Verification items for the finished model (mm, model axes). A direction names the side the tool comes from. Round coordinates to 2 decimals unless told otherwise and drop trailing zeros. Write each loop counter-clockwise with the first axis right and the second up, starting at its lowest first coordinate (ties: lowest second). Pieces come first, ordered by that corner, then holes. Notation, with made-up numbers: (53, -24) - (107, -24) arc R20 ccw to (107, 10) - close; hole circle Ø6 at (12.25, -7). An arc over 180 degrees is marked (long way). Answer as a JSON object with one key per item and string values.
```python
from build123d import *

# Parameters (mm, degrees)
SKETCH1_R           = 7
BOSS_EXTRUDE1_DEPTH = 4
SKETCH2_R           = 7
SKETCH2_R_2         = 5
BOSS_EXTRUDE2_DEPTH = 10
BOSS_EXTRUDE3_DEPTH = 10
BOSS_EXTRUDE4_DEPTH = 9
FILLET3_R           = 1.35
CHAMFER1_SIZE       = 2.7
SKETCH7_R           = 1.5
CUT_EXTRUDE1_DEPTH  = 10
FILLET4_R           = 2
SKETCH8_R           = 0.5
CUT_EXTRUDE2_DEPTH  = 25.534299997


# Some blends are built 0.0001 mm under size
with BuildPart() as part:
    # Sketch1 → Boss-Extrude1 (new body)
    with BuildSketch(Plane.XY):
        Circle(SKETCH1_R)
    extrude(amount=BOSS_EXTRUDE1_DEPTH)

    # Sketch2 → Boss-Extrude2 (add)
    with BuildSketch(Plane.XY.offset(4)):
        Circle(SKETCH2_R)
        Circle(SKETCH2_R_2, mode=Mode.SUBTRACT)
    extrude(amount=BOSS_EXTRUDE2_DEPTH)

    # Sketch3 → Boss-Extrude3 (add)
    with BuildSketch(Plane.XY.offset(4)):
        with BuildLine():
            Line((-1.35, 4.814301611), (-1.35, -4.814301611))
            ThreePointArc((-1.35, -4.814301611), (-5, 0), (-1.35, 4.814301611))
        make_face()
        with BuildLine():
            Line((1.35, 4.814301611), (1.35, -4.814301611))
            ThreePointArc((1.35, -4.814301611), (5, 0), (1.35, 4.814301611))
        make_face()
    extrude(amount=BOSS_EXTRUDE3_DEPTH)

    # Sketch4 → Boss-Extrude4 (add)
    with BuildSketch(Plane(origin=(0, 0, 0), x_dir=(-1, 0, 0), z_dir=(0, 0, -1))):
        with BuildLine():
            Line((2.05, 0), (4.242640687, 0))
            Line((4.242640687, 0), (10.242640687, 0))
            Line((10.242640687, 0), (10.242640687, -1.5))
            Line((10.242640687, -1.5), (4.242640687, -1.5))
            ThreePointArc((4.242640687, -1.5), (0, -4.5), (-4.242640687, -1.5))
            Line((-4.242640687, -1.5), (-10.242640687, -1.5))
            Line((-10.242640687, -1.5), (-10.242640687, 0))
            Line((-10.242640687, 0), (-4.242640687, 0))
            Line((-4.242640687, 0), (-2.05, 0))
            ThreePointArc((-2.05, 0), (0, -2.05), (2.05, 0))
        make_face()
    extrude(amount=BOSS_EXTRUDE4_DEPTH)

    # Fillet3
    fillet3_edges = [part.edges().sort_by_distance(p)[0] for p in [
        (-1.35, 4.814301611, 9),
    ]]
    fillet(fillet3_edges, radius=FILLET3_R)
    fillet3_2_edges = [part.edges().sort_by_distance(p)[0] for p in [
        (1.35, 4.814301611, 9),
    ]]
    fillet(fillet3_2_edges, radius=FILLET3_R - 0.0001)  # a hair under: the kernel refuses the full size
    fillet3_3_edges = [part.edges().sort_by_distance(p)[0] for p in [
        (1.35, -4.814301611, 9),
    ]]
    fillet(fillet3_3_edges, radius=FILLET3_R)
    fillet3_4_edges = [part.edges().sort_by_distance(p)[0] for p in [
        (-1.35, -4.814301611, 9),
    ]]
    fillet(fillet3_4_edges, radius=FILLET3_R - 0.0001)  # a hair under: the kernel refuses the full size
    fillet3_5_edges = [part.edges().sort_by_distance(p)[0] for p in [
        (-1.35, -4.9999e-05, 4),
    ]]
    fillet(fillet3_5_edges, radius=FILLET3_R - 0.0001)  # a hair under: the kernel refuses the full size

    # Chamfer1
    # the kernel refuses this chamfer: 2.7 mm, written as the material it adds along each edge
    with BuildSketch(Plane(origin=(0, 0, 0), x_dir=(-1, 0, 0), z_dir=(0, 1, 0))) as chamfer1_piece_1_section:
        Polygon((7, CHAMFER1_SIZE), (7 + CHAMFER1_SIZE, 0), (7, 0), align=None)
    chamfer1_piece_1 = revolve(axis=Axis((0, 0, 0), (0, 0, 1)), revolution_arc=69.20773796, mode=Mode.PRIVATE)
    chamfer1_piece_1 = split(chamfer1_piece_1, bisect_by=Plane(origin=(-7.851109484, -1.5, 0.900303531), z_dir=(0, 1, 0)), keep=Keep.TOP, mode=Mode.PRIVATE)
    add(chamfer1_piece_1)
    with BuildSketch(Plane(origin=(0, 0, 0), x_dir=(0.3549807082679851, -0.9348736260894087, 0), z_dir=(-0.9348736260894087, -0.3549807082679851, 0))) as chamfer1_piece_2_section:
        Polygon((7, CHAMFER1_SIZE), (7 + CHAMFER1_SIZE, 0), (7, 0), align=None)
    chamfer1_piece_2 = revolve(axis=Axis((0, 0, 0), (0, 0, 1)), revolution_arc=69.20773796, mode=Mode.PRIVATE)
    chamfer1_piece_2 = split(chamfer1_piece_2, bisect_by=Plane(origin=(7.851109484, -1.5, 0.900303531), z_dir=(0, 1, 0)), keep=Keep.TOP, mode=Mode.PRIVATE)
    add(chamfer1_piece_2)

    # Sketch7 → Cut-Extrude1 (cut)
    with BuildSketch(Plane(origin=(0, 0, 0), x_dir=(1, 0, 0), z_dir=(0, 1, 0))):
        with Locations(Location((7.242640687, 4.5, 0), (0, 0, 180))):
            Circle(SKETCH7_R)
        with Locations(Location((-7.242640687, 4.5, 0), (0, 0, 180))):
            Circle(SKETCH7_R)
    extrude(amount=-CUT_EXTRUDE1_DEPTH, mode=Mode.SUBTRACT)

    # Fillet4
    fillet4_edges = [part.edges().sort_by_distance(p)[0] for p in [
        (-6.837397166, -1.5, 1.35),
        (6.837397166, -1.5, 1.35),
        (-5.540018926, -1.5, 0),
        (5.540018926, -1.5, 0),
        (0, -4.5, 0),
    ]]
    fillet(fillet4_edges, radius=FILLET4_R)

    # Sketch8 → Cut-Extrude2 (cut, through all)
    with BuildSketch(Plane(origin=(8.65, 0, 0), x_dir=(0, 0, -1), z_dir=(1, 0, 0))):
        with Locations((-12.5, 0)):
            Circle(SKETCH8_R)
    extrude(amount=-CUT_EXTRUDE2_DEPTH, mode=Mode.SUBTRACT)


solid = part.part
```
1. Material ranges on probe 1 along X at (y, z) = (3, 8); probe 2 along X at (y, z) = (-2.5, 11); probe 3 along Y at (x, z) = (4.15, 12.5), recorded low to high. Write a range as from..to.
Completed:
{"probe 1": "x = -6.32..-1.35, 1.35..6.32", "probe 2": "x = -6.54..-1.35, 1.35..6.54", "probe 3": "y = -5.64..-0.5, 0.5..5.64"}
2. Cross-section at A-A (z = -4.5). Record the boundary of the cut face in (x, y).
Completed:
{"outline": "(-10.24, -1.5) - (-8.74, -1.5) - (-8.74, 0) - (-10.24, 0) - close; (-5.74, -1.5) - (-4.24, -1.5) arc R4.5 ccw to (4.24, -1.5) - (5.74, -1.5) - (5.74, 0) - (2.05, 0) arc R2.05 cw to (-2.05, 0) - (-5.74, 0) - close; (8.74, -1.5) - (10.24, -1.5) - (10.24, 0) - (8.74, 0) - close"}
3. Cross-section at D-D (y = -1). Count the separate pieces of the cut face and the enclosed holes in it, plus the area to 3 significant figures.
Completed:
{"separate pieces": "1", "enclosed holes": "2", "area": "313 mm^2"}
4. Access from +Z, -Z, +X, -X, +Y, -Y to the whole of each face (thin tool, end or side, straight path). Record for faces 1 (the face through (0.97, 0.05, 4.41)), 2 (the face through (-4, 0, 13)), 3 (the face through (5.85, -1.85, -0.87)), 4 (the face through (-7.2, -1.5, -6.2)).
Completed:
{"face 1": "+Z", "face 2": "+X, -X", "face 3": "-Z, +X, -Y", "face 4": "-Z, -X, -Y"}
5. Go/stop test with flat-tipped pins: pin 1 (4 mm diameter, centred on x = -3.5, z = -1, fed in from -Y); pin 2 (2 mm diameter, centred on y = 5.5, z = 2, fed in from -X); pin 3 (3 mm diameter, centred on x = 7, z = -5.5, fed in from -Y). Record where each tip stops, or that it passes through.
Completed:
{"pin 1": "stops at y = -6.77", "pin 2": "stops at x = -5.36", "pin 3": "stops at y = -1.5"}
6. Mould release check, pull along X, two halves, no side actions. Record for faces 5 (the face through (-0.1, -4.5, -5.5)), 6 (the face through (-0.97, 4.59, 9.74)), 7 (the face through (0, -6.7, 0)): released by +X, released by -X, zero draft, split by the parting line, or undercut.
Completed:
{"face 5": "split by the parting line", "face 6": "undercut", "face 7": "zero draft"}
